Here's how the part is built. I have some questions about the finished solid (model axes, mm). A direction names the side the tool comes from. Coordinates: 2 decimals unless noted, no trailing zeros. Loops run counter-clockwise (first coordinate to the right, second up) from the corner with the lowest first, then second, coordinate; pieces in that order, holes last.
```python
from build123d import *

# Parameters (mm, degrees)
F0_R     = 10.16
F1_DEPTH = 38.1
F2_W     = 25.4
F2_H     = 25.4
F3_DEPTH = 2.54


with BuildPart() as f1:
    # F0 (on Top) → F1 (new body)
    with BuildSketch(Plane.XY):
        Circle(F0_R)
    extrude(amount=F1_DEPTH)

    # F2 (on Top) → F3 (join)
    with BuildSketch(Plane.XY):
        Rectangle(F2_W, F2_H)
    extrude(amount=F3_DEPTH)


solid = f1.part
```
1. I need wall thicknesses on line 1 along Y through (x, z) = (0, 4.5); line 2 along Z through (x, y) = (-10.75, -6.25). Which ranges of each line are inside material? Lowest first, please.
2. On a 3-axis mill with a long thin cutter (end or side, diameter ignored), from which of +Z, -Z, +X, -X, +Y, -Y can I reach the whole of each face in a straight line? I mean faces 1 (the flat face through (12.7, 0, 1)), 2 (the flat face through (-6, 9, 2.54)). Say none if no direction works.
3. I want a section at C-C (z = 17). Please give me the cut outline in (x, y).
4. I want a section at A-A (y = 0). Please give me the cut outline in (x, z).
5. For pin 1 (10 mm diameter, centred on y = 4.5, z = 14.5, fed in from -X); pin 2 (6 mm diameter, centred on y = 10, z = 31, fed in from -X); pin 3 (3 mm diameter, centred on y = -6.5, z = 11, fed in from -X), each with a flat end and sliding along its axis, tell me the tip position at first contact or that it passes through.
Response values:
1. line 1: y = -10.16 to 10.16
1. line 2: z = 0 to 2.54
2. face 1: +Z, -Z, +X, +Y, -Y
2. face 2: +Z
3. outline: circle Ø20.32 at (0, 0)
4. outline: (-12.7, 0) - (12.7, 0) - (12.7, 2.54) - (10.16, 2.54) - (10.16, 38.1) - (-10.16, 38.1) - (-10.16, 2.54) - (-12.7, 2.54) - close
5. pin 1: stops at x = -10.16
5. pin 2: stops at x = -7.36
5. pin 3: stops at x = -8.84
